Input: dimensioned drawing with shaded views. Units: mm. Origin: part minimum x, y, z. A direction names the side the tool comes from. Round coordinates to 2 decimals unless told otherwise and drop trailing zeros. Loops run counter-clockwise (first coordinate to the right, second up) from the corner with the lowest first, then second, coordinate; pieces in that order, holes last. Notation, with made-up numbers: (20, 67.5) - (42, 67.5) arc R36 ccw to (42, 103.5) - close; hole circle Ø1 at (10.5, 50.5). An arc over 180 degrees is marked (long way). One line per question, with ' | ' between items. Start each with the question number.
Item 1: Section C-C, the plane z = 9.75. Return loops of the section in (x, y), plus the area to 3 significant figures.
Item 2: Set-up query: the marked faces 1, 2, 3, 4 and 5. Return all of +Z, -Z, +X, -X, +Y, -Y with unobstructed straight access to the full face (end or side cutting, diameter ignored); none if empty.
Item 3: Section B-B, the plane x = 124.5. Return loops of the section in (y, z), plus the area to 3 significant figures.
Item 4: Section A-A, the plane y = 4.75. Return loops of the section in (x, z).
Item 5: First-contact query: pin 1 (0.8 mm diameter, centred on y = 7, z = 1.5, fed in from +X); pin 2 (2 mm diameter, centred on y = 6.5, z = 10, fed in from -X); pin 3 (2.5 mm diameter, centred on y = 5.5, z = 10, fed in from +X). Flat tips, straight axial feed; report the tip coordinate or a pass-through.
Item 6: Material intervals for line 1 along Z through (x, y) = (122.5, 8.5); line 2 along Z through (x, y) = (78, 6.25); line 3 along X through (y, z) = (4.25, 5.5), sorted ascending.
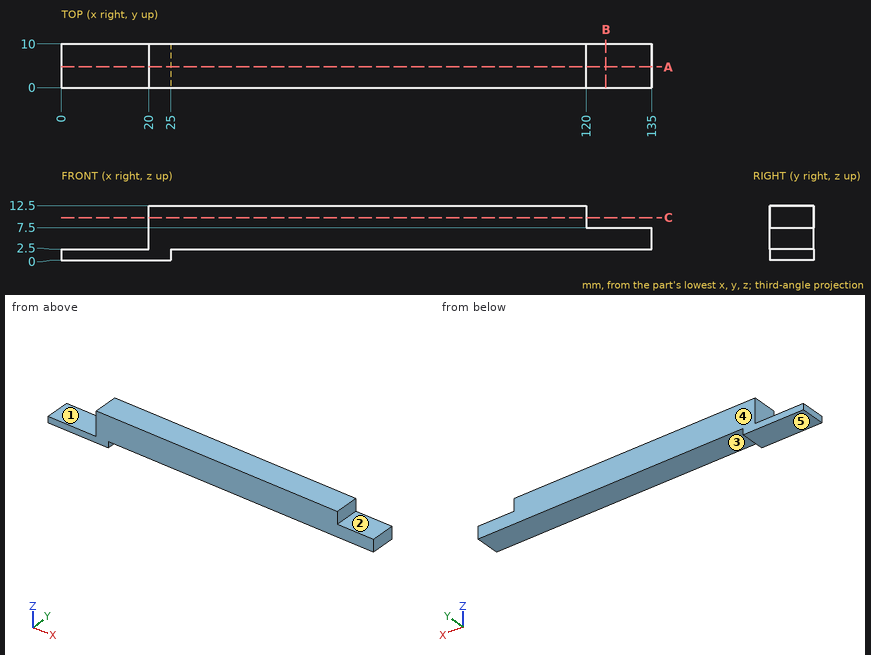
Return value:
1) outline: (20, 0) - (120, 0) - (120, 10) - (20, 10) - close | area: 1,000 mm2
2) face 1: +Z, -X, +Y, -Y | face 2: +Z, +X, +Y, -Y | face 3: -Z, +X, +Y, -Y | face 4: +Z, -Z, +X, -X, +Y | face 5: -Z, +X, -X, +Y, -Y
3) outline: (0, 2.5) - (10, 2.5) - (10, 7.5) - (0, 7.5) - close | area: 50.0 mm2
4) outline: (0, 0) - (25, 0) - (25, 2.5) - (135, 2.5) - (135, 7.5) - (120, 7.5) - (120, 12.5) - (20, 12.5) - (20, 2.5) - (0, 2.5) - close
5) pin 1: x = 25 | pin 2: x = 20 | pin 3: x = 120
6) line 1: 2.5 to 7.5 | line 2: 2.5 to 12.5 | line 3: 20 to 135
